Model file for the job. Use its own axes, mm. Give positions to 0.01 mm unless a question says otherwise; leave off trailing zeros. Loops run counter-clockwise (first coordinate to the right, second up) from the corner with the lowest first, then second, coordinate; pieces in that order, holes last. Notation, with made-up numbers: (-12, 31) - (10, 31) arc R25 ccw to (10, 53) - close; hole circle Ø3 at (-39.75, 82.5). An arc over 180 degrees is marked (long way). Use a Markdown table: item, result.
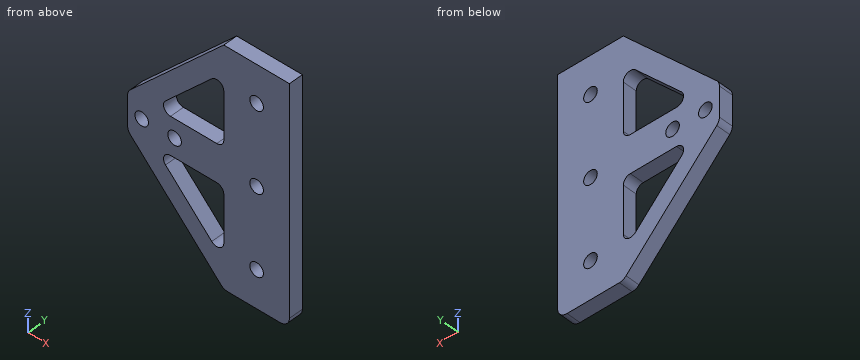
from build123d import *

# Parameters (mm, degrees)
EXTRUDE_1_DEPTH     = 3
SKETCH_2_W          = 14
SKETCH_2_H          = 50
EXTRUDE_2_DEPTH     = 3
SKETCH_3_R          = 1.45
CUT_EXTRUDE_1_DEPTH = 46.169126624
EXTRUDE_3_DEPTH     = 3
FILLET_1_R          = 1.5
FILLET_2_R          = 2


with BuildPart() as part:
    # 草图1 → 凸台-拉伸1 (new body)
    with BuildSketch(Plane(origin=(0, 0, 0), x_dir=(1, 0, 0), z_dir=(0, 1, 0))):
        with BuildLine():
            ThreePointArc((8.55, 4), (10, 5.45), (11.45, 4))
            Line((11.45, 4), (27.5, 4))
            Line((27.5, 4), (27.5, 8))
            Line((27.5, 8), (0, 8))
            Line((0, 8), (0, 4))
            Line((0, 4), (1.55, 4))
            ThreePointArc((1.55, 4), (3, 5.45), (4.45, 4))
            Line((4.45, 4), (8.55, 4))
        make_face()
        with BuildLine():
            Line((27.5, 4), (11.45, 4))
            ThreePointArc((11.45, 4), (10, 2.55), (8.55, 4))
            Line((8.55, 4), (4.45, 4))
            ThreePointArc((4.45, 4), (3, 2.55), (1.55, 4))
            Line((1.55, 4), (0, 4))
            Line((0, 4), (0, 0))
            Line((0, 0), (27.5, 0))
            Line((27.5, 0), (27.5, 4))
        make_face()
    extrude(amount=EXTRUDE_1_DEPTH)

    # 草图2 → 凸台-拉伸2 (add)
    with BuildSketch(Plane(origin=(0, 3, 0), x_dir=(1, 0, 0), z_dir=(0, 1, 0))):
        with Locations((27.5, 4)):
            Rectangle(SKETCH_2_W, SKETCH_2_H)
    extrude(amount=-EXTRUDE_2_DEPTH)

    # 草图3 → 切除-拉伸1 (cut, through all)
    with BuildSketch(Plane(origin=(0, 3, 0), x_dir=(1, 0, 0), z_dir=(0, 1, 0))):
        with Locations(Location((27.5, 21, 0), (0, 0, 270))):
            Circle(SKETCH_3_R)
        with Locations(Location((27.5, 4, 0), (0, 0, 270))):
            Circle(SKETCH_3_R)
        with Locations(Location((27.5, -13, 0), (0, 0, 270))):
            Circle(SKETCH_3_R)
    extrude(amount=-CUT_EXTRUDE_1_DEPTH, mode=Mode.SUBTRACT)

    # 草图4 → 凸台-拉伸3 (add)
    with BuildSketch(Plane(origin=(0, 3, 0), x_dir=(1, 0, 0), z_dir=(0, 1, 0))):
        Polygon((0, 8), (20.5, 29), (20.5, 23.27374416), (5.589916416, 8), align=None)
        Polygon((20.5, -21), (0, 0), (5.589916416, 0), (20.5, -15.27374416), align=None)
    extrude(amount=-EXTRUDE_3_DEPTH)

    # 圆角1
    fillet_1_edges = [part.edges().sort_by_distance(p)[0] for p in [
        (20.5, 1.5, 0),
        (20.5, 1.5, -8),
        (5.589916416, 1.5, -8),
        (20.5, 1.5, -23.27374416),
        (20.5, 1.5, 15.27374416),
        (5.589916416, 1.5, 0),
    ]]
    fillet(fillet_1_edges, radius=FILLET_1_R)

    # 圆角2
    fillet_2_edges = [part.edges().sort_by_distance(p)[0] for p in [
        (0, 1.5, -8),
        (0, 1.5, 0),
        (20.5, 1.5, -29),
        (34.5, 1.5, -29),
    ]]
    fillet(fillet_2_edges, radius=FILLET_2_R)


solid = part.part
(1) Slice it at B-B, the plane z = -4. Write the cut outline in (x, y), plus the area to 3 significant figures.
Computed:
| item | result |
|---|---|
| outline | (0, 0) - (1.55, 0) - (1.55, 3) - (0, 3) - close; (4.45, 0) - (8.55, 0) - (8.55, 3) - (4.45, 3) - close; (11.45, 0) - (26.05, 0) - (26.05, 3) - (11.45, 3) - close; (28.95, 0) - (34.5, 0) - (34.5, 3) - (28.95, 3) - close |
| area | 77.4 mm² |
(2) Drill centre lines: probe 1 along Z at (x, y) = (14, 2.3); probe 2 along Z at (x, y) = (8, 1.4); probe 3 along X at (y, z) = (1.8, -3). Where is each one in solid material? Low to high. Write a range as [from, to].
Computed:
| item | result |
|---|---|
| probe 1 | [-22.34, -16.62], [-8, 0], [8.62, 14.34] |
| probe 2 | [-16.2, -10.46], [-8.54, 0.54], [2.46, 8.2] |
| probe 3 | [0, 1.95], [4.05, 8.95], [11.05, 26.45], [28.55, 34.5] |
(3) Slice it at A-A, the plane x = 27.5. Write the cut outline in (y, z), plus the area to 3 significant figures.
Computed:
| item | result |
|---|---|
| outline | (0, -29) - (3, -29) - (3, -22.45) - (0, -22.45) - close; (0, -19.55) - (3, -19.55) - (3, -5.45) - (0, -5.45) - close; (0, -2.55) - (3, -2.55) - (3, 11.55) - (0, 11.55) - close; (0, 14.45) - (3, 14.45) - (3, 21) - (0, 21) - close |
| area | 124 mm² |
(4) Pin check, flat tips, straight feed: P1, Ø1, axis at y = 0.5, z = -16.5, coming from the -X side; P2, Ø4.5, axis at x = 3, z = -4, coming from the +Y side. Stop position of each tip, or through.
Computed:
| item | result |
|---|---|
| P1 | x = 7.81 |
| P2 | y = 3 |
(5) Slice it at C-C, the plane y = 1.45. Write the cut outline in (x, z), plus the area to 3 significant figures.
Computed:
| item | result |
|---|---|
| outline | (0, -7.19) arc R2 ccw to (0.57, -8.58) - (19.91, -28.4) arc R2 ccw to (21.34, -29) - (32.5, -29) arc R2 ccw to (34.5, -27) - (34.5, 21) - (20.5, 21) - (0.57, 0.58) arc R2 ccw to (0, -0.81) - close; hole circle Ø2.9 at (3, -4); hole (8.08, -10.55) - (17.93, -20.64) arc R1.5 ccw to (20.5, -19.59) - (20.5, -9.5) arc R1.5 ccw to (19, -8) - (9.15, -8) arc R1.5 ccw to start; hole (8.08, 2.55) arc R1.5 ccw to (9.15, 0) - (19, 0) arc R1.5 ccw to (20.5, 1.5) - (20.5, 11.59) arc R1.5 ccw to (17.93, 12.64) - close; hole circle Ø2.9 at (10, -4); hole circle Ø2.9 at (27.5, -21); hole circle Ø2.9 at (27.5, -4); hole circle Ø2.9 at (27.5, 13) |
| area | 1,040 mm² |
(6) Slice it at D-D, the plane x = 3. Write the cut outline in (y, z), plus the area to 3 significant figures.
Computed:
| item | result |
|---|---|
| outline | (0, -11.07) - (3, -11.07) - (3, -5.45) - (0, -5.45) - close; (0, -2.55) - (3, -2.55) - (3, 3.07) - (0, 3.07) - close |
| area | 33.7 mm² |
